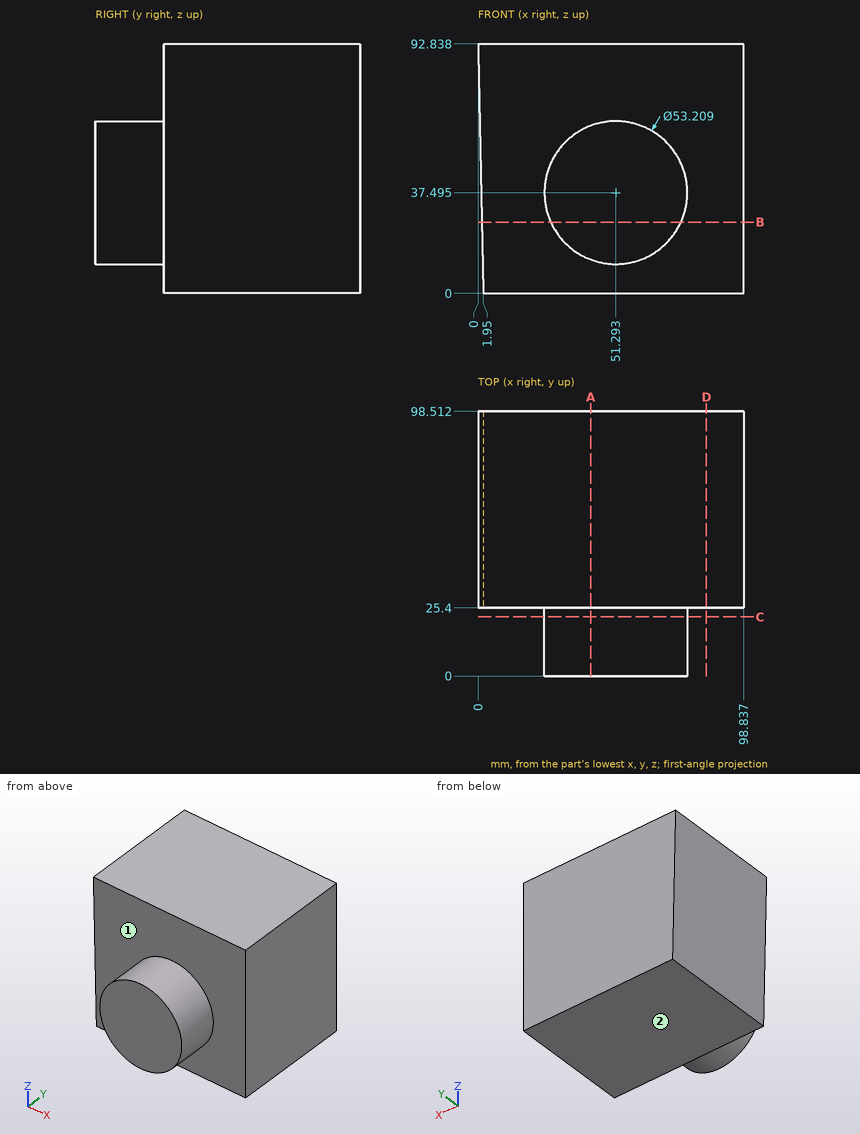
The drawing under review shows one solid part. Ordinate dimensions are in mm from its lowest x, y, z. A direction names the side the tool comes from. Round coordinates to 2 decimals unless told otherwise and drop trailing zeros. Write each loop counter-clockwise with the first axis right and the second up, starting at its lowest first coordinate (ties: lowest second). Pieces come first, ordered by that corner, then holes. Notation, with made-up numbers: M 43.5,-11 L 60.5,-11 A9 cw 60.5,1 Z; hole C 29,24 d1. An arc over 180 degrees is marked long. One line per item, written item: value. Start each with the question number.
(1) Machinability: for the marked faces 1 and 2, which of the approach directions +Z, -Z, +X, -X, +Y, -Y give a long, thin tool a straight path to every point of the face, cutting with its end or side? Answer none if there is none.
(2) We need section A-A (x = 42). Give the boundary of the cut face in (y, z), and give its area (3 significant figures).
(3) We need section C-C (y = 22). Give the boundary of the cut face in (x, z) (1 decimal).
(4) Wall thickness on line 1 (Y direction, x = 42, z = 75.5); line 2 (X direction, y = 75, z = 56.5); line 3 (X direction, y = 73, z = 38): over which ranges is each line inside the solid? List them lowest first.
(5) We need section D-D (x = 85). Give the boundary of the cut face in (y, z), and give its area (3 significant figures).
(6) Insertion check: pin 1 (1.5 mm diameter, centred on y = 59.5, z = 11, fed in from -X); pin 2 (12 mm diameter, centred on x = 57, z = 60, fed in from -Y); pin 3 (3 mm diameter, centred on x = 77, y = 21, fed in from +Z) (1 decimal); pin 4 (8 mm diameter, centred on x = 82, z = 65, fed in from -Y). Each pin has a flat end and moves straight along its axis. Give the tip position at first contact, or say it passes through.
(7) We need section B-B (z = 26.5). Give the boundary of the cut face in (x, y).
Result:
1. face 1: -Y
1. face 2: -Z, +X, -X, +Y, -Y
2. outline: M 0,12.57 L 25.4,12.57 L 25.4,0 L 98.51,0 L 98.51,92.84 L 25.4,92.84 L 25.4,62.42 L 0,62.42 Z
2. area: 8,050 mm²
3. outline: C 51.3,37.5 d53.2
4. line 1: 25.4 to 98.51
4. line 2: 0.76 to 98.84
4. line 3: 1.15 to 98.84
5. outline: M 25.4,0 L 98.51,0 L 98.51,92.84 L 25.4,92.84 Z
5. area: 6,790 mm²
6. pin 1: x = 1.7
6. pin 2: y = 0
6. pin 3: z = 48.5
6. pin 4: y = 25.4
7. outline: M 1.39,25.4 L 27.07,25.4 L 27.07,0 L 75.52,0 L 75.52,25.4 L 98.84,25.4 L 98.84,98.51 L 1.39,98.51 Z
